Check sheet for the modelled part. Datum: model origin and axes. Units: mm. Give positions to 0.01 mm unless a question says otherwise; leave off trailing zeros. Order: outer loops, then holes, each group sorted by start corner. A loop starts at its lowest first (then second) coordinate and runs counter-clockwise, first axis right, second up. Notation, with made-up numbers: M 1.5,65 L 54.5,65 A27 cw 54.5,96 Z; hole C 11.25,71.25 d4. An arc over 180 degrees is marked long. Return JSON: item names as keys, results as strings. Group by question number.
from build123d import *

# Parameters (mm, degrees)
SKETCH1_W             = 152.4
SKETCH1_H             = 20
BOSS_EXTRUDE1_DEPTH   = 3.175
F_6_CLEARANCE_HOLE1_D = 3.7973


with BuildPart() as part:
    # Sketch1 → Boss-Extrude1 (new body)
    with BuildSketch(Plane.XY):
        with Locations((76.2, 10)):
            Rectangle(SKETCH1_W, SKETCH1_H)
    extrude(amount=BOSS_EXTRUDE1_DEPTH)

    # #6 Clearance Hole1 (through all)
    with Locations(Plane(origin=(0, 0, 0), x_dir=(-1, 0, 0), z_dir=(0, 0, -1))):
        with Locations((-142.4, 10), (-10, 10)):
            Hole(F_6_CLEARANCE_HOLE1_D / 2)


solid = part.part
1) Depth check by flat-ended pin: P1, Ø3.5, axis at x = 10, y = 10, coming from the -Z side. Enter the tip coordinate at first touch or a pass-through.
2) Release check for a two-part mould opening along Y. For faces 1 (the face through (0, 10, 2)), 2 (the face through (9.753, 11.882, 1.61)), 3 (the face through (75, 0, 2)) record: released by +Y, released by -Y, zero draft, split by the parting line, or undercut.
3) Material ranges on line 1 along X through (y, z) = (11.5, 0.3); line 2 along Y through (x, z) = (142.4, 1.45); line 3 along Y through (x, z) = (143, 3), recorded low to high.
4) Sectioned sample at A-A on x = 10. Record the boundary of the cut face in (y, z) (3 decimals).
5) Sectioned sample at B-B on y = 10. Record the boundary of the cut face in (x, z) (3 decimals).
Reply:
{
 "1": {"P1": "through"},
 "2": {"face 1": "zero draft", "face 2": "undercut", "face 3": "released by -Y"},
 "3": {"line 1": "0 to 8.84, 11.16 to 141.24, 143.56 to 152.4", "line 2": "0 to 8.1, 11.9 to 20", "line 3": "0 to 8.2, 11.8 to 20"},
 "4": {"outline": "M 0,0 L 8.101,0 L 8.101,3.175 L 0,3.175 Z; M 11.899,0 L 20,0 L 20,3.175 L 11.899,3.175 Z"},
 "5": {"outline": "M 0,0 L 8.101,0 L 8.101,3.175 L 0,3.175 Z; M 11.899,0 L 140.501,0 L 140.501,3.175 L 11.899,3.175 Z; M 144.299,0 L 152.4,0 L 152.4,3.175 L 144.299,3.175 Z"}
}
